```python
from build123d import *

# Parameters (mm, degrees)
SKETCH1_R           = 1.5
BOSS_EXTRUDE1_DEPTH = 2
SKETCH3_R           = 30
CUT_EXTRUDE1_DEPTH  = 147.410555656
M3_5_TAPPED_HOLE1_D = 2.9


with BuildPart() as part:
    # Sketch1 → Boss-Extrude1 (new body)
    with BuildSketch(Plane(origin=(0, 0, 0), x_dir=(1, 0, 0), z_dir=(0, 1, 0))):
        with BuildLine():
            ThreePointArc((-92.04043234, 41.60778152), (-73.883899315, -0.003033538), (-92.04602482, -41.611407917))
            ThreePointArc((-92.04602482, -41.611407917), (-95.261127604, -55.002885894), (-82.053611962, -58.905461822))
            ThreePointArc((-82.053611962, -58.905461822), (-36.939322536, -63.986850506), (-9.986476067, -100.51989977))
            ThreePointArc((-9.986476067, -100.51989977), (0.003332664, -109.999999445), (9.986820378, -100.513243342))
            ThreePointArc((9.986820378, -100.513243342), (36.944576778, -63.983816968), (82.059548754, -58.908491853))
            ThreePointArc((82.059548754, -58.908491853), (95.264460267, -54.997113551), (92.04043234, -41.60778152))
            ThreePointArc((92.04043234, -41.60778152), (73.883899315, 0.003033538), (92.04602482, 41.611407917))
            ThreePointArc((92.04602482, 41.611407917), (95.261127604, 55.002885894), (82.053611962, 58.905461822))
            ThreePointArc((82.053611962, 58.905461822), (36.939322536, 63.986850506), (9.986476067, 100.51989977))
            ThreePointArc((9.986476067, 100.51989977), (-0.003332664, 109.999999445), (-9.986820378, 100.513243342))
            ThreePointArc((-9.986820378, 100.513243342), (-36.944576778, 63.983816968), (-82.059548754, 58.908491853))
            ThreePointArc((-82.059548754, 58.908491853), (-95.264460267, 54.997113551), (-92.04043234, 41.60778152))
        make_face()
        with Locations(Location((86.602540378, 50, 0), (0, 0, 90))):
            Circle(SKETCH1_R, mode=Mode.SUBTRACT)
        with Locations(Location((86.602540378, -50, 0), (0, 0, 90))):
            Circle(SKETCH1_R, mode=Mode.SUBTRACT)
        with Locations(Location((0, -100, 0), (0, 0, 90))):
            Circle(SKETCH1_R, mode=Mode.SUBTRACT)
        with Locations(Location((-86.602540378, -50, 0), (0, 0, 90))):
            Circle(SKETCH1_R, mode=Mode.SUBTRACT)
        with Locations(Location((-86.602540378, 50, 0), (0, 0, 90))):
            Circle(SKETCH1_R, mode=Mode.SUBTRACT)
        with Locations(Location((0, 100, 0), (0, 0, 90))):
            Circle(SKETCH1_R, mode=Mode.SUBTRACT)
        with Locations(Location((-25, 43.301270189, 0), (0, 0, 90))):
            Circle(SKETCH1_R, mode=Mode.SUBTRACT)
        with Locations(Location((25, 43.301270189, 0), (0, 0, 90))):
            Circle(SKETCH1_R, mode=Mode.SUBTRACT)
        with Locations(Location((50, 0, 0), (0, 0, 90))):
            Circle(SKETCH1_R, mode=Mode.SUBTRACT)
        with Locations(Location((25, -43.301270189, 0), (0, 0, 90))):
            Circle(SKETCH1_R, mode=Mode.SUBTRACT)
        with Locations(Location((-50, 0, 0), (0, 0, 90))):
            Circle(SKETCH1_R, mode=Mode.SUBTRACT)
        with Locations(Location((-25, -43.301270189, 0), (0, 0, 90))):
            Circle(SKETCH1_R, mode=Mode.SUBTRACT)
    extrude(amount=BOSS_EXTRUDE1_DEPTH)

    # Sketch3 → Cut-Extrude1 (cut, through all)
    with BuildSketch(Plane(origin=(0, 0, 0), x_dir=(-1, 0, 0), z_dir=(0, -1, 0))):
        with Locations(Location((0, 0, 0), (0, 0, 90))):
            Circle(SKETCH3_R)
    extrude(amount=-CUT_EXTRUDE1_DEPTH, mode=Mode.SUBTRACT)

    # M3.5 Tapped Hole1 (through all)
    with Locations(Plane(origin=(-25.4, 2, -34.29), x_dir=(0, 0, 1), z_dir=(0, 1, 0))):
        with Locations((0, 0), (0, 50.8), (68.58, 50.8), (68.58, 0)):
            Hole(M3_5_TAPPED_HOLE1_D / 2)


solid = part.part
```
Can you work these out from the model? Positions are in its coordinate system, mm. Coordinates: 2 decimals unless noted, no trailing zeros. Loops run counter-clockwise (first coordinate to the right, second up) from the corner with the lowest first, then second, coordinate; pieces in that order, holes last. Notation, with made-up numbers: (87.5, 2) - (108.5, 2) arc R13 ccw to (108.5, 11) - close; hole circle Ø7 at (-1.5, 51.25). An arc over 180 degrees is marked (long way). Answer as CSV lines item,"result". Start each with the question number.
1) Suppose I cut it at D-D (z = -83). Please give me the cut outline in (x, y).
2) Suppose I cut it at C-C (x = 58.5). Please give me the cut outline in (y, z), plus the area to 3 significant figures.
3) I need wall thicknesses on line 1 (X direction, y = 0.75, z = 0); line 2 (Z direction, x = 25, y = 0.6); line 3 (X direction, y = 1.6, z = 50). Which ranges of each line are inside material? Lowest first, please. Write a range as from..to.
4) For pin 1 (2.5 mm diameter, centred on x = 50, z = 0, fed in from -Y); pin 2 (4 mm diameter, centred on x = 25, z = -43.3, fed in from -Y), each with a flat end and sliding along its axis, tell me the tip position at first contact or that it passes through.
5) Thinking about a two-plate mould opening in X: for faces 1 (the cylindrical face through (-73.888, 0.986, -0.651)), 2 (the cylindrical face through (73.888, 0.986, 0.651)), 3 (the cylindrical face through (37.51, 0.99, -63.66)), which applies, pulls with the +X half, pulls with the -X half, needs draft (parallel to the pull), parting line crosses it, or undercut?
6) Suppose I cut it at B-B (y = 0.4). Count the separate pieces of the cut face and the enclosed holes in it, plus the area to 3 significant figures.
7) Suppose I cut it at A-A (z = 12). Please give me the cut outline in (x, y), plus the area to 3 significant figures.
Check result:
1,outline,"(-17.23, 0) - (17.23, 0) - (17.23, 2) - (-17.23, 2) - close"
2,outline,"(0, -56.79) - (2, -56.79) - (2, 56.79) - (0, 56.79) - close"
2,area,"227 mm²"
3,line 1,"x = -73.88..-51.5, -48.5..-30, 30..48.5, 51.5..73.88"
3,line 2,"z = -73.19..-44.8, -41.8..-35.68, -32.9..-16.58, 16.58..32.9, 35.68..41.8, 44.8..73.19"
3,line 3,"x = -96.6..-88.1, -85.1..85.1, 88.1..96.6"
4,pin 1,"passes through"
4,pin 2,"stops at y = 0"
5,face 1,"pulls with the -X half"
5,face 2,"pulls with the +X half"
5,face 3,"undercut"
6,separate pieces,"1"
6,enclosed holes,"17"
6,area,"20,700 mm²"
7,outline,"(-75.17, 0) - (-27.5, 0) - (-27.5, 2) - (-75.17, 2) - close; (27.5, 0) - (75.17, 0) - (75.17, 2) - (27.5, 2) - close"
7,area,"191 mm²"
